Part model, mm, in its own coordinate system. Face numbers are marked on the shaded views. A direction names the side the tool comes from. Coordinates: 2 decimals unless noted, no trailing zeros. Order: outer loops, then holes, each group sorted by start corner. A loop starts at its lowest first (then second) coordinate and runs counter-clockwise, first axis right, second up.
1) Wall check: L1, parallel to Z at x = 0, y = -12.6; L2, parallel to X at y = -5, z = -5.5; L3, parallel to Y at x = 0, z = 16. Give the ranges that are in metal, low to high.
2) Cut at B-B (y = -4.25). Give the number of separate pieces and of enclosed holes in the cut face, and give its area (3 significant figures).
3) Mould opens along Y. For the marked faces 1, 2, 3 and 4 say: +Y half, -Y half, draft (parallel to the pull), parting line (faces both ways), or undercut.
4) Tool access for the marked faces 5 and 6: list every direction of +Z, -Z, +X, -X, +Y, -Y with a clear straight run to the whole face (end or side of a thin tool).
5) Pin check, flat tip, straight feed: pin 1 Ø1.3 at (x, z) = (-28, -2.5) entering from -Y. Stop position of the tip, or through.
6) Cut at A-A (x = -23.5). List the corners of the cut face in (y, z), and give its area (3 significant figures).
```python
from build123d import *

# Parameters (mm, degrees)
SKETCH_W        = 60
SKETCH_H        = 29.5
PAD_DEPTH       = 20
SKETCH020_R     = 1.7
SKETCH020_R_2   = 14
POCKET_DEPTH    = 20
SKETCH001_R     = 1.75
SKETCH001_R_2   = 4.5
POCKET001_DEPTH = 5
SKETCH024_R     = 2.220567
PAD001_DEPTH    = 4
POCKET003_DEPTH = 6
SKETCH022_R     = 2
POCKET004_DEPTH = 3
SKETCH023_W     = 7
SKETCH023_H     = 4.2
POCKET005_DEPTH = 1.6
CHAMFER_SIZE    = 1
CHAMFER001_SIZE = 1
CHAMFER002_SIZE = 1.5
CHAMFER003_SIZE = 1.5
CHAMFER004_SIZE = 1.5
CHAMFER005_SIZE = 1.5
FILLET_R        = 4
FILLET001_R     = 4
FILLET002_R     = 2
FILLET003_R     = 2
FILLET004_R     = 2
FILLET005_R     = 2


with BuildPart() as part:
    # Sketch → Pad (new body, symmetric)
    with BuildSketch(Plane.XY):
        Rectangle(SKETCH_W, SKETCH_H)
        Polygon((-27, -7.75), (-12.5, -11.75), (12.5, -11.75), (27, -7.75), (27, 8.25), (10, 11.25), (-10, 11.25), (-27, 8.25), align=None, mode=Mode.SUBTRACT)
    extrude(amount=PAD_DEPTH, both=True)

    # Sketch020 → Pocket (cut)
    with BuildSketch(Plane(origin=(0, 14.75, 0), x_dir=(-1, 0, 0), z_dir=(0, 1, 0))):
        with Locations((-17.320508, 10)):
            Circle(SKETCH020_R)
        with Locations((-17.320508, -10)):
            Circle(SKETCH020_R)
        with Locations((17.320508, 10)):
            Circle(SKETCH020_R)
        with Locations((17.320508, -10)):
            Circle(SKETCH020_R)
        Circle(SKETCH020_R_2)
    extrude(amount=-POCKET_DEPTH, mode=Mode.SUBTRACT)

    # Sketch001 → Pocket001 (cut)
    with BuildSketch(Plane.XZ.offset(14.75)):
        with Locations((0, 8)):
            Circle(SKETCH001_R)
        with Locations((0, -8)):
            Circle(SKETCH001_R)
        with Locations((-9.5, 0)):
            Circle(SKETCH001_R)
        with Locations((9.5, 0)):
            Circle(SKETCH001_R)
        Circle(SKETCH001_R_2)
    extrude(amount=-POCKET001_DEPTH, mode=Mode.SUBTRACT)

    # Sketch024 → Pad001 (new body)
    with BuildSketch(Plane.XZ.offset(-11.25)):
        with Locations((-17.320508, 10)):
            Circle(SKETCH024_R)
    extrude(amount=PAD001_DEPTH)

    # Sketch021 → Pocket003 (cut)
    with BuildSketch(Plane.XZ.offset(-7.25)):
        Polygon((-18.937089, 12.8), (-20.55367, 10), (-18.937089, 7.2), (-15.703927, 7.2), (-14.087347, 10), (-15.703927, 12.8), align=None)
        Polygon((15.703927, 12.8), (14.087347, 10), (15.703927, 7.2), (18.937089, 7.2), (20.55367, 10), (18.937089, 12.8), align=None)
        Polygon((-18.937089, -7.2), (-20.55367, -10), (-18.937089, -12.8), (-15.703927, -12.8), (-14.087347, -10), (-15.703927, -7.2), align=None)
        Polygon((15.703927, -7.2), (14.087347, -10), (15.703927, -12.8), (18.937089, -12.8), (20.55367, -10), (18.937089, -7.2), align=None)
    extrude(amount=-POCKET003_DEPTH, mode=Mode.SUBTRACT)

    # Sketch022 → Pocket004 (cut)
    with BuildSketch(Plane(origin=(-30, 0, 0), x_dir=(0, -1, 0), z_dir=(-1, 0, 0))):
        with Locations((3, 3.13)):
            Circle(SKETCH022_R)
        with Locations((3, -3.13)):
            Circle(SKETCH022_R)
    extrude(amount=-POCKET004_DEPTH, mode=Mode.SUBTRACT)

    # Sketch023 → Pocket005 (cut)
    with BuildSketch(Plane.YZ.offset(-27)):
        with Locations((0.5, 3.13)):
            Rectangle(SKETCH023_W, SKETCH023_H)
        with Locations((0.5, -3.13)):
            Rectangle(SKETCH023_W, SKETCH023_H)
    extrude(amount=-POCKET005_DEPTH, mode=Mode.SUBTRACT)

    # Chamfer
    chamfer_edges = [part.edges().sort_by_distance(p)[0] for p in [
        (-30, -1, 3.13),
    ]]
    chamfer(chamfer_edges, length=CHAMFER_SIZE)

    # Chamfer001
    chamfer001_edges = [part.edges().sort_by_distance(p)[0] for p in [
        (-30, -1, -3.13),
    ]]
    chamfer(chamfer001_edges, length=CHAMFER001_SIZE)

    # Chamfer002
    chamfer002_edges = [part.edges().sort_by_distance(p)[0] for p in [
        (-1.75, -14.75, 8),
    ]]
    chamfer(chamfer002_edges, length=CHAMFER002_SIZE)

    # Chamfer003
    chamfer003_edges = [part.edges().sort_by_distance(p)[0] for p in [
        (-11.25, -14.75, 0),
    ]]
    chamfer(chamfer003_edges, length=CHAMFER003_SIZE)

    # Chamfer004
    chamfer004_edges = [part.edges().sort_by_distance(p)[0] for p in [
        (7.75, -14.75, 0),
    ]]
    chamfer(chamfer004_edges, length=CHAMFER004_SIZE)

    # Chamfer005
    chamfer005_edges = [part.edges().sort_by_distance(p)[0] for p in [
        (-1.75, -14.75, -8),
    ]]
    chamfer(chamfer005_edges, length=CHAMFER005_SIZE)

    # Fillet
    fillet_edges = [part.edges().sort_by_distance(p)[0] for p in [
        (-30, -14.75, 0),
    ]]
    fillet(fillet_edges, radius=FILLET_R)

    # Fillet001
    fillet001_edges = [part.edges().sort_by_distance(p)[0] for p in [
        (30, -14.75, 0),
    ]]
    fillet(fillet001_edges, radius=FILLET001_R)

    # Fillet002
    fillet002_edges = [part.edges().sort_by_distance(p)[0] for p in [
        (-27, 8.25, 0),
    ]]
    fillet(fillet002_edges, radius=FILLET002_R)

    # Fillet003
    fillet003_edges = [part.edges().sort_by_distance(p)[0] for p in [
        (27, 8.25, 0),
    ]]
    fillet(fillet003_edges, radius=FILLET003_R)

    # Fillet004
    fillet004_edges = [part.edges().sort_by_distance(p)[0] for p in [
        (-27, -7.75, 0),
    ]]
    fillet(fillet004_edges, radius=FILLET004_R)

    # Fillet005
    fillet005_edges = [part.edges().sort_by_distance(p)[0] for p in [
        (27, -7.75, 0),
    ]]
    fillet(fillet005_edges, radius=FILLET005_R)


solid = part.part
```
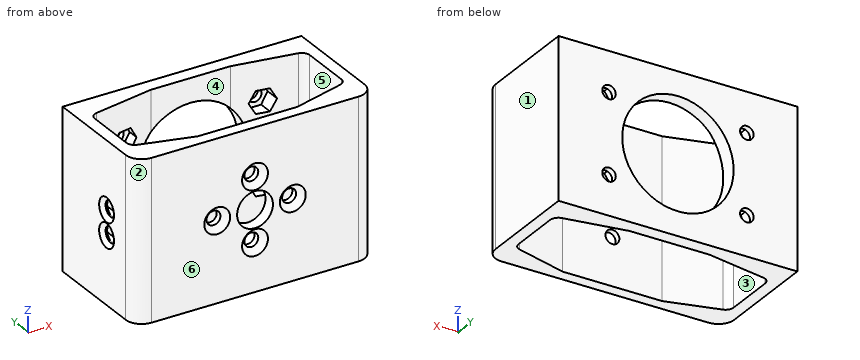
Geometry check:
1. L1: z = -20 to -9.75, -6.25 to -4.5, 4.5 to 6.25, 9.75 to 20
1. L2: x = -30 to -27, 27 to 30
1. L3: y = -14.75 to -11.75, 11.25 to 14.75
2. separate pieces: 4
2. enclosed holes: 0
2. area: 219 mm2
3. face 1: draft
3. face 2: -Y half
3. face 3: undercut
3. face 4: undercut
4. face 5: +Z, -Z
4. face 6: +Z, -Z, +X, -X, -Y
5. pin 1: stops at y = -14.52
6. outline: (-14.75, -20) - (-8.72, -20) - (-8.72, 20) - (-14.75, 20) - close; (8.87, -20) - (14.75, -20) - (14.75, 20) - (8.87, 20) - close
6. area: 477 mm2
